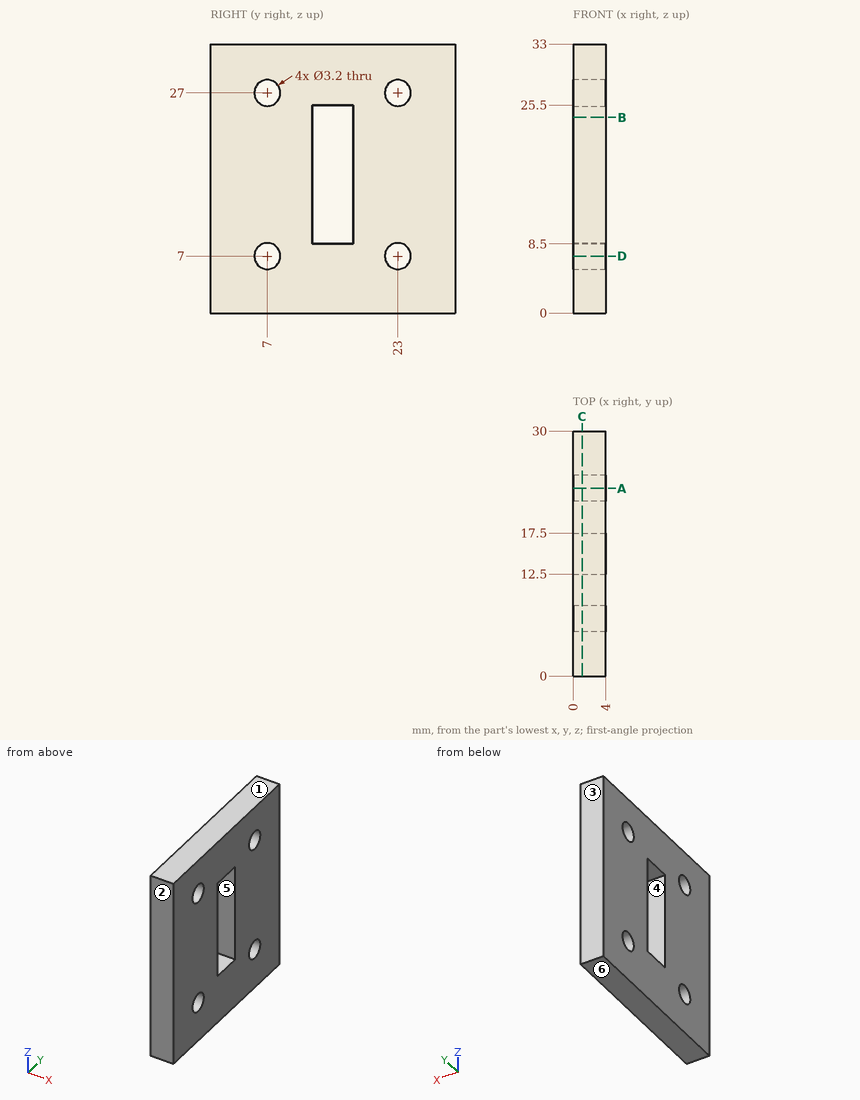
Part print with two shaded views. Sizes in mm from the minimum x, y, z corner. A direction names the side the tool comes from. Round coordinates to 2 decimals unless told otherwise and drop trailing zeros. Order: outer loops, then holes, each group sorted by start corner. A loop starts at its lowest first (then second) coordinate and runs counter-clockwise, first axis right, second up. Notation, with made-up numbers: (-30, 34.25) - (-25, 34.25) arc R30 cw to (-25, 62.25) - close; hole circle Ø4 at (51, -33.5). An arc over 180 degrees is marked (long way). Answer as CSV lines item,"result". Start each with the question number.
1. Drill centre lines: L1, parallel to Y at x = 3.2, z = 7; L2, parallel to Y at x = 1.7, z = 12; L3, parallel to Z at x = 1.4, y = 24. Where is each one in solid material? Low to high. Write a range as [from, to].
2. Tool access for the marked faces 5 and 6: list every direction of +Z, -Z, +X, -X, +Y, -Y with a clear straight run to the whole face (end or side of a thin tool).
3. Saw through at D-D, the plane z = 7. Write the cut outline in (x, y).
4. Saw through at A-A, the plane y = 23. Write the cut outline in (x, z), and give its area (3 significant figures).
5. Saw through at B-B, the plane z = 24. Write the cut outline in (x, y).
6. Saw through at C-C, the plane x = 1.1. Write the cut outline in (y, z).
7. Pull direction Y, two halves, no side cores. Call the marked faces 1, 2, 3 and 4: +Y half, -Y half, draft (parallel to the pull), parting line (faces both ways), or undercut.
Model answer:
1,L1,"y = [0, 5.4], [8.6, 21.4], [24.6, 30]"
1,L2,"y = [0, 12.5], [17.5, 30]"
1,L3,"z = [0, 5.75], [8.25, 25.75], [28.25, 33]"
2,face 5,"+X, -X"
2,face 6,"-Z, +X, -X, +Y, -Y"
3,outline,"(0, 0) - (4, 0) - (4, 5.4) - (0, 5.4) - close; (0, 8.6) - (4, 8.6) - (4, 21.4) - (0, 21.4) - close; (0, 24.6) - (4, 24.6) - (4, 30) - (0, 30) - close"
4,outline,"(0, 0) - (4, 0) - (4, 5.4) - (0, 5.4) - close; (0, 8.6) - (4, 8.6) - (4, 25.4) - (0, 25.4) - close; (0, 28.6) - (4, 28.6) - (4, 33) - (0, 33) - close"
4,area,"106 mm²"
5,outline,"(0, 0) - (4, 0) - (4, 12.5) - (0, 12.5) - close; (0, 17.5) - (4, 17.5) - (4, 30) - (0, 30) - close"
6,outline,"(0, 0) - (30, 0) - (30, 33) - (0, 33) - close; hole circle Ø3.2 at (7, 7); hole circle Ø3.2 at (7, 27); hole (12.5, 8.5) - (17.5, 8.5) - (17.5, 25.5) - (12.5, 25.5) - close; hole circle Ø3.2 at (23, 7); hole circle Ø3.2 at (23, 27)"
7,face 1,"draft"
7,face 2,"-Y half"
7,face 3,"+Y half"
7,face 4,"undercut"
